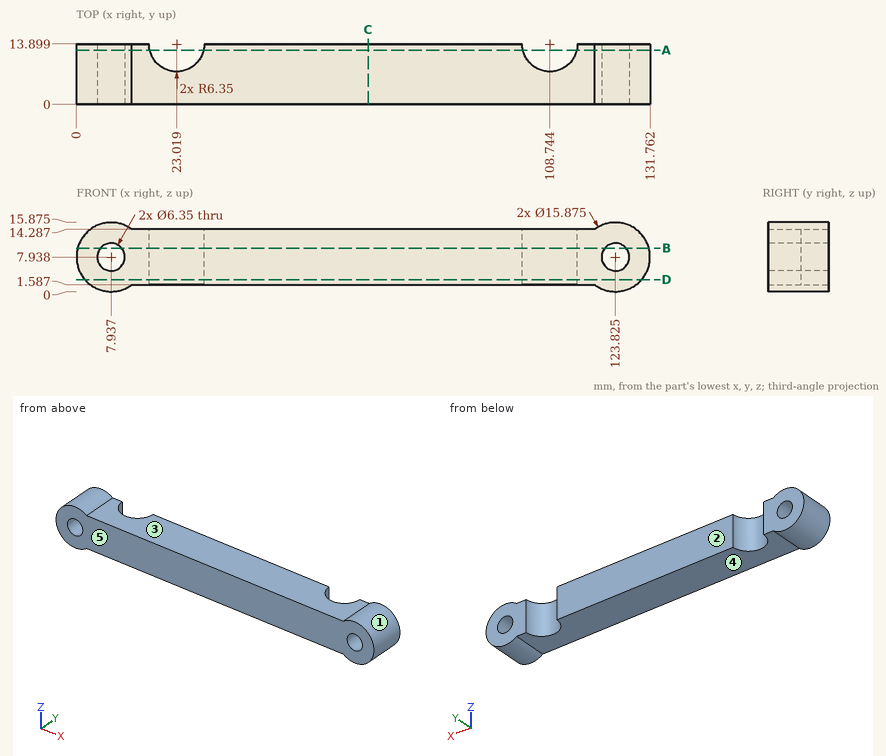
Can you work these out from the drawing? Everything is in mm from the part's minimum corner. A direction names the side the tool comes from. Round coordinates to 2 decimals unless told otherwise and drop trailing zeros. Order: outer loops, then holes, each group sorted by start corner. A loop starts at its lowest first (then second) coordinate and runs counter-clockwise, first axis right, second up. Notation, with made-up numbers: (56, -9.75) -> (105, -9.75) arc R22 cw to (105, 1.25) -> close; hole circle Ø9 at (30.25, 49.25). An arc over 180 degrees is marked (long way). Use CSV: the item, a comma, the result in double quotes.
1. I want a section at B-B on z = 10. List the corners of the cut face in (x, y) for me.
Recorded:
outline,"(0.27, 0) -> (5.52, 0) -> (5.52, 13.9) -> (0.27, 13.9) -> close; (10.35, 0) -> (121.41, 0) -> (121.41, 13.9) -> (115.09, 13.9) arc R6.35 cw to (102.39, 13.9) -> (29.37, 13.9) arc R6.35 cw to (16.67, 13.9) -> (10.35, 13.9) -> close; (126.24, 0) -> (131.49, 0) -> (131.49, 13.9) -> (126.24, 13.9) -> close"
2. I need wall thicknesses on line 1 along X through (y, z) = (6.75, 7.75) (1 decimal); line 2 along X through (y, z) = (3.5, 9.25) (1 decimal); line 3 along Z through (x, y) = (106, 7). Which ranges of each line are inside material? Lowest first, please.
Recorded:
line 1,"x = 0 to 4.8, 11.1 to 120.7, 127 to 131.8"
line 2,"x = 0.1 to 5, 10.8 to 120.9, 126.7 to 131.7"
line 3,"z = 1.59 to 14.29"
3. I'm going to push flat-ended pins straight in: P1, Ø2, axis at y = 11.5, z = 10.5, coming from the -X side (1 decimal); P2, Ø1, axis at x = 61, y = 9.5, coming from the -Z side; P3, Ø1, axis at y = 3, z = 9.5, coming from the -X side. Where does each tip first touch, or does it pass through?
Recorded:
P1,"stops at x = 0.2"
P2,"stops at z = 1.59"
P3,"stops at x = 0.07"
4. Which directions (+Z, -Z, +X, -X, +Y, -Y) give clear straight access to the entire face, cutting with the end or side of a thin tool? Please do the marked faces 3, 4 and 5.
Recorded:
face 3,"+Z, +Y, -Y"
face 4,"-Z, +Y, -Y"
face 5,"+Z, -Z, +X, -X, -Y"
5. Thinking about a two-plate mould opening in X: for the marked faces 1 and 2, which applies, pulls with the +X half, pulls with the -X half, needs draft (parallel to the pull), parting line crosses it, or undercut?
Recorded:
face 1,"undercut"
face 2,"needs draft"
6. I want a section at D-D on z = 2.75. List the corners of the cut face in (x, y) for me.
Recorded:
outline,"(1.93, 0) -> (129.83, 0) -> (129.83, 13.9) -> (115.09, 13.9) arc R6.35 cw to (102.39, 13.9) -> (29.37, 13.9) arc R6.35 cw to (16.67, 13.9) -> (1.93, 13.9) -> close"
7. I want a section at A-A on y = 12.5. Give the number of separate pieces and of enclosed holes in the cut face, and give its area (3 significant figures).
Recorded:
separate pieces,"3"
enclosed holes,"2"
area,"1,310 mm2"
8. I want a section at C-C on x = 67. List the corners of the cut face in (y, z) for me.
Recorded:
outline,"(0, 1.59) -> (13.9, 1.59) -> (13.9, 14.29) -> (0, 14.29) -> close"
